The listing builds one solid part. Answer for the finished solid, in the listing's coordinates (mm). A direction names the side the tool comes from. Round coordinates to 2 decimals unless told otherwise and drop trailing zeros. Write each loop counter-clockwise with the first axis right and the second up, starting at its lowest first coordinate (ties: lowest second). Pieces come first, ordered by that corner, then holes. Notation, with made-up numbers: (1.25, 37) - (59.25, 37) arc R15 cw to (59.25, 63) - close; hole circle Ø10 at (49.5, 36). An arc over 180 degrees is marked (long way). Answer in a Markdown table with one row per item.
from build123d import *

# Parameters (mm, degrees)
SKETCH1_W                        = 88.9
SKETCH1_H                        = 88.9
BOSS_EXTRUDE1_DEPTH              = 19.05
SKETCH2_R                        = 38.1
CUT_EXTRUDE1_DEPTH               = 16.51
F_10_32_TAPPED_HOLE1_AT_2_COUNT  = 2
F_10_32_TAPPED_HOLE1_AT_2_PITCH  = 76.2
F_10_32_TAPPED_HOLE2_D           = 4.0386
F_10_32_TAPPED_HOLE2_DEPTH       = 14.986
F_10_32_TAPPED_HOLE2_CBORE_D     = 4.826
F_10_32_TAPPED_HOLE2_CBORE_DEPTH = 12.7
F_10_32_TAPPED_HOLE2_TIP         = 1.213317848


with BuildPart() as part:
    # Sketch1 → Boss-Extrude1 (new body)
    with BuildSketch(Plane.XY):
        Rectangle(SKETCH1_W, SKETCH1_H)
    extrude(amount=BOSS_EXTRUDE1_DEPTH)

    # Sketch2 → Cut-Extrude1 (cut)
    with BuildSketch(Plane.XY.offset(19.05)):
        Circle(SKETCH2_R)
    extrude(amount=-CUT_EXTRUDE1_DEPTH, mode=Mode.SUBTRACT)

    # Sketch3 → #10-32 Tapped Hole1 (revolve, cut)
    with BuildSketch(Plane(origin=(-38.1, 44.45, 9.525), x_dir=(0, 0, 1), z_dir=(1, 0, 0))):
        Polygon((0, 0), (0, 22.640757848), (2.0193, 21.42744), (2.0193, 19.05), (2.413, 19.05), (2.413, 0), align=None)
    f_10_32_tapped_hole1 = revolve(axis=Axis((-38.1, 50.8, 9.525), (0, -1, 0)), mode=Mode.SUBTRACT)

    # #10-32 Tapped Hole1 at 2: #10-32 Tapped Hole1 ×2
    with Locations(*[(i * F_10_32_TAPPED_HOLE1_AT_2_PITCH, 0, 0) for i in range(1, F_10_32_TAPPED_HOLE1_AT_2_COUNT)]):
        add(f_10_32_tapped_hole1, mode=Mode.SUBTRACT)

    # Mirror1: #10-32 Tapped Hole1 across plane
    add(f_10_32_tapped_hole1.mirror(Plane.ZX), mode=Mode.SUBTRACT)

    # Mirror1 copy 1 sketch → Mirror1 copy 1 (revolve, cut)
    with BuildSketch(Plane(origin=(38.1, -44.45, 9.525), x_dir=(0, 0, 1), z_dir=(1, 0, 0))):
        Polygon((0, 0), (0, -22.640757848), (2.0193, -21.42744), (2.0193, -19.05), (2.413, -19.05), (2.413, 0), align=None)
    revolve(axis=Axis((38.1, -50.8, 9.525), (0, -1, 0)), mode=Mode.SUBTRACT)

    # #10-32 Tapped Hole2
    with Locations(Plane.XY.offset(19.05)):
        with Locations((30.48, -30.48), (-30.48, -30.48), (-30.48, 30.48), (30.48, 30.48)):
            CounterBoreHole(F_10_32_TAPPED_HOLE2_D / 2, F_10_32_TAPPED_HOLE2_CBORE_D / 2, F_10_32_TAPPED_HOLE2_CBORE_DEPTH, depth=F_10_32_TAPPED_HOLE2_DEPTH)
            with Locations((0, 0, -(F_10_32_TAPPED_HOLE2_DEPTH + F_10_32_TAPPED_HOLE2_TIP / 2))):  # 118° drill point
                Cone(0, F_10_32_TAPPED_HOLE2_D / 2, F_10_32_TAPPED_HOLE2_TIP, mode=Mode.SUBTRACT)


solid = part.part
(1) For faces 5 (the cylindrical face through (-39.803, 24.228, 10.611)), 6 (the flat face through (44.45, -1, 9)), 7 (the cylindrical face through (29.548, -32.271, 5.191)), determine the directions among +Z, -Z, +X, -X, +Y, -Y from which every point of the face is accessible in a straight line to the end or side of a thin tool.
Checked values:
| item | result |
|---|---|
| face 5 | +Y |
| face 6 | +Z, -Z, +X, +Y, -Y |
| face 7 | +Z |
(2) Section A-A (z = 13.5) is taken. Give the vertices of the cut face in (x, y), and give its area (3 significant figures).
Checked values:
| item | result |
|---|---|
| outline | (-44.45, -44.45) - (44.45, -44.45) - (44.45, 44.45) - (-44.45, 44.45) - close; hole circle Ø76.2 at (0, 0); hole circle Ø4.83 at (-30.48, -30.48); hole circle Ø4.83 at (-30.48, 30.48); hole circle Ø4.83 at (30.48, -30.48); hole circle Ø4.83 at (30.48, 30.48) |
| area | 3,270 mm2 |
(3) Flat-ended cylindrical pins translate along their axes: pin 1 (3.5 mm diameter, centred on x = 30.48, y = -30.48, fed in from +Z); pin 2 (3 mm diameter, centred on x = -38.1, z = 9.525, fed in from -Y); pin 3 (4.5 mm diameter, centred on x = 38.1, z = 9.525, fed in from -Y). Find the tip coordinate at first contact, or state that the pin passes through.
Checked values:
| item | result |
|---|---|
| pin 1 | stops at z = 3.9 |
| pin 2 | stops at y = -22.71 |
| pin 3 | stops at y = -25.4 |
(4) For a pull along Z with two mould halves and no side action, classify faces 1 (the flat face through (-1, -44.45, 9)), 2 (the flat face through (-1, 1, 2.54)), 3 (the cylindrical face through (39.024, -35.058, 11.754)), 4 (the conical face through (37.8, 22.02, 9.71)) as pulls with the +Z half, pulls with the -Z half, needs draft (parallel to the pull), parting line crosses it, or undercut.
Checked values:
| item | result |
|---|---|
| face 1 | needs draft |
| face 2 | pulls with the +Z half |
| face 3 | undercut |
| face 4 | undercut |
(5) Find the intervals of material crossed by line 1 (Y direction, x = 30.48, z = 10); line 2 (X direction, y = 33, z = 11); line 3 (Z direction, x = -25, y = -13.5), in increasing order.
Checked values:
| item | result |
|---|---|
| line 1 | y = -44.45 to -32.89, -28.07 to -22.86, 22.86 to 28.07, 32.89 to 44.45 |
| line 2 | x = -44.45 to -40.01, -36.19 to -19.04, 19.04 to 36.19, 40.01 to 44.45 |
| line 3 | z = 0 to 2.54 |
(6) Section B-B (x = 0) is taken. Give the vertices of the cut face in (y, z).
Checked values:
| item | result |
|---|---|
| outline | (-44.45, 0) - (44.45, 0) - (44.45, 19.05) - (38.1, 19.05) - (38.1, 2.54) - (-38.1, 2.54) - (-38.1, 19.05) - (-44.45, 19.05) - close |
(7) Section C-C (y = 1.5) is taken. Give the vertices of the cut face in (x, z).
Checked values:
| item | result |
|---|---|
| outline | (-44.45, 0) - (44.45, 0) - (44.45, 19.05) - (38.07, 19.05) - (38.07, 2.54) - (-38.07, 2.54) - (-38.07, 19.05) - (-44.45, 19.05) - close |
